Model file for the job. Use its own axes, mm. A direction names the side the tool comes from. Coordinates: 2 decimals unless noted, no trailing zeros. Order: outer loops, then holes, each group sorted by start corner. A loop starts at its lowest first (then second) coordinate and runs counter-clockwise, first axis right, second up.
from build123d import *

# Parameters (mm, degrees)
F1_R     = 28.575
F2_DEPTH = 40.2336
F3_R     = 3.302
F4_DEPTH = 40.2336
F7_DEPTH = 15.7734
F5_R     = 10.16
F8_DEPTH = 25.4


with BuildPart() as f2:
    # F1 (on Top) → F2 (new body)
    with BuildSketch(Plane.XY):
        Circle(F1_R)
    extrude(amount=F2_DEPTH)

    # F3
    f3_edges = [f2.edges().sort_by_distance(p)[0] for p in [
        (-28.575, 0, 40.2336),
    ]]
    fillet(f3_edges, radius=F3_R)

    # F0 (on Top) → F4 (cut)
    with BuildSketch(Plane.XY):
        with BuildLine():
            Line((8.8773, 0), (14.2875, 0))
            ThreePointArc((14.2875, 0), (13.8739387677, 3.4126938508), (12.6571966832, 6.6278222948))
            Line((12.6571966832, 6.6278222948), (8.8773, 6.6278222948))
            Line((8.8773, 6.6278222948), (8.8773, 0))
        make_face()
        with BuildLine():
            Line((18.5293, 0), (14.2875, 0))
            ThreePointArc((14.2875, 0), (13.6943674733, -4.0739361504), (11.9642166044, -7.8096208163))
            Line((11.9642166044, -7.8096208163), (18.5293, -7.8096208163))
            Line((18.5293, -7.8096208163), (18.5293, 0))
        make_face()
        with BuildLine():
            ThreePointArc((12.6571966832, 6.6278222948), (13.8739387677, 3.4126938508), (14.2875, 0))
            Line((14.2875, 0), (18.5293, 0))
            Line((18.5293, 0), (18.5293, 6.6278222948))
            Line((18.5293, 6.6278222948), (12.6571966832, 6.6278222948))
        make_face()
        with BuildLine():
            ThreePointArc((11.9642166044, -7.8096208163), (13.6943674733, -4.0739361504), (14.2875, 0))
            Line((14.2875, 0), (8.8773, 0))
            Line((8.8773, 0), (8.8773, -7.8096208163))
            Line((8.8773, -7.8096208163), (11.9642166044, -7.8096208163))
        make_face()
        with BuildLine():
            Line((8.8773, 6.6278222948), (12.6571966832, 6.6278222948))
            ThreePointArc((12.6571966832, 6.6278222948), (-3.4126938508, 13.8739387677), (-14.2875, 0))
            Line((-14.2875, 0), (8.8773, 0))
            Line((8.8773, 0), (8.8773, 6.6278222948))
        make_face()
        with BuildLine():
            ThreePointArc((-14.2875, 0), (-4.0739361504, -13.6943674733), (11.9642166044, -7.8096208163))
            Line((11.9642166044, -7.8096208163), (8.8773, -7.8096208163))
            Line((8.8773, -7.8096208163), (8.8773, 0))
            Line((8.8773, 0), (-14.2875, 0))
        make_face()
    extrude(amount=F4_DEPTH, mode=Mode.SUBTRACT)

    # F6 (on Top) → F7 (join)
    with BuildSketch(Plane.XY):
        Polygon((36.9937829673, -19.6861159056), (36.9937829673, 19.4048862904), (51.9836863995, 19.4048862904), (0, 28.4042526037), (21.5210951865, 10.1242884994), (21.5210951865, -8.7181376293), (0, -28.6854840815), (51.9836863995, -19.6861159056), align=None)
        with BuildLine():
            Line((51.9836863995, 19.4048862904), (36.9937829673, 19.4048862904))
            Line((36.9937829673, 19.4048862904), (36.9937829673, -19.6861159056))
            Line((36.9937829673, -19.6861159056), (51.9836863995, -19.6861159056))
            ThreePointArc((51.9836863995, -19.6861159056), (65.4540705811, -14.1065000872), (71.0336863995, -0.6361159056))
            Line((71.0336863995, -0.6361159056), (71.0336863995, 0.3548862904))
            ThreePointArc((71.0336863995, 0.3548862904), (65.4540705811, 13.825270472), (51.9836863995, 19.4048862904))
        make_face()
    extrude(amount=F7_DEPTH)

    # F5 (on Top) → F8 (cut)
    with BuildSketch(Plane.XY):
        with Locations((53.975, 0)):
            Circle(F5_R)
    extrude(amount=F8_DEPTH, mode=Mode.SUBTRACT)


solid = f2.part
Q1. Probe line 1 (Z direction, x = 45, y = 18); line 2 (Y direction, x = 6, z = 25); line 3 (X direction, y = -12, z = 10.5). List the from-to ranges inside material, lowest first.
Established:
line 1: z = 0 to 15.77
line 2: y = -27.94 to -12.97, 12.97 to 27.94
line 3: x = -25.93 to -7.75, 7.75 to 67.27
Q2. Mould opens along Y. For faces 3 (the face through (-28.547, 1.256, 22.311)), 4 (the face through (21, 0, 0)), 5 (the face through (43.825, 0.447, 7.776)) say: pulls with the +Y half, pulls with the -Y half, needs draft (parallel to the pull), parting line crosses it, or undercut.
Established:
face 3: parting line crosses it
face 4: needs draft
face 5: undercut
Q3. Drop flat-ended pins along their axis: P1, Ø6, axis at y = 12, z = 34, coming from the -X side; P2, Ø18.5, axis at x = 53.975, y = 0, coming from the -Z side; P3, Ø8, axis at x = 40.5, y = -13, coming from the +Z side; P4, Ø11.5, axis at y = -2.5, z = 25, coming from the -X side (3 decimals). Give the stop position or say it passes through.
Established:
P1: stops at x = -27.12
P2: passes through
P3: stops at z = 15.77
P4: stops at x = -28.575
Q4. Which spindle directions (+Z, -Z, +X, -X, +Y, -Y) get a long thin tool onto all of the face, cutting with end or side? Do faces 1 (the face through (65.6, 13.68, 7.78)), 2 (the face through (15, -7.81, 20)). Say none if no direction does.
Established:
face 1: +Z, -Z, +X, +Y
face 2: +Z, -Z
Q5. Cut at A-A, the plane z = 12. Count the separate pieces of the cut face and the enclosed holes in it, plus the area to 3 significant figures.
Established:
separate pieces: 1
enclosed holes: 2
area: 3,340 mm2
Q6. Cut at B-B, the plane x = 58.5. List the corners of the cut face in (y, z).
Established:
outline: (-18.54, 0) - (-9.1, 0) - (-9.1, 15.77) - (-18.54, 15.77) - close; (9.1, 0) - (18.26, 0) - (18.26, 15.77) - (9.1, 15.77) - close
